Check sheet for the drawn part. Datum: minimum x, y, z corner. Units: mm. A direction names the side the tool comes from. Coordinates: 2 decimals unless noted, no trailing zeros. Order: outer loops, then holes, each group sorted by start corner. A loop starts at its lowest first (then second) coordinate and runs counter-clockwise, first axis right, second up. Notation, with made-up numbers: M 9,22.25 L 44,22.25 A31 cw 44,59.25 Z; hole C 83,78.25 d10. An arc over 180 degrees is marked long. Return JSON: item names as keys, results as strings. Group by question number.
Q1. Section check C-C, the plane x = 30. Enter the section's corners in (y, z), then the cut area to 3 significant figures.
Q2. Access from +Z, -Z, +X, -X, +Y, -Y to the whole of each face (thin tool, end or side, straight path). Record for the marked faces 1 and 2.
Q3. Go/stop test with flat-tipped pins: pin 1 Ø3.5 at (y, z) = (42, 6.5) entering from -X; pin 2 Ø3.5 at (y, z) = (39, 6) entering from +X. Record where each tip stops, or that it passes through.
Q4. Section check D-D, the plane y = 54.5. Enter the section's corners in (x, z), then the cut area to 3 significant figures.
Q5. Thickness scan on probe 1 along X at (y, z) = (22, 1.75); probe 2 along Z at (x, y) = (50, 20); probe 3 along X at (y, z) = (25.5, 8.25). Record the ranges inside material, lowest first.
Q6. Section check B-B, the plane y = 21. Enter the section's corners in (x, z).
Q7. Section check A-A, the plane z = 9. Enter the section's corners in (x, y), then the cut area to 3 significant figures.
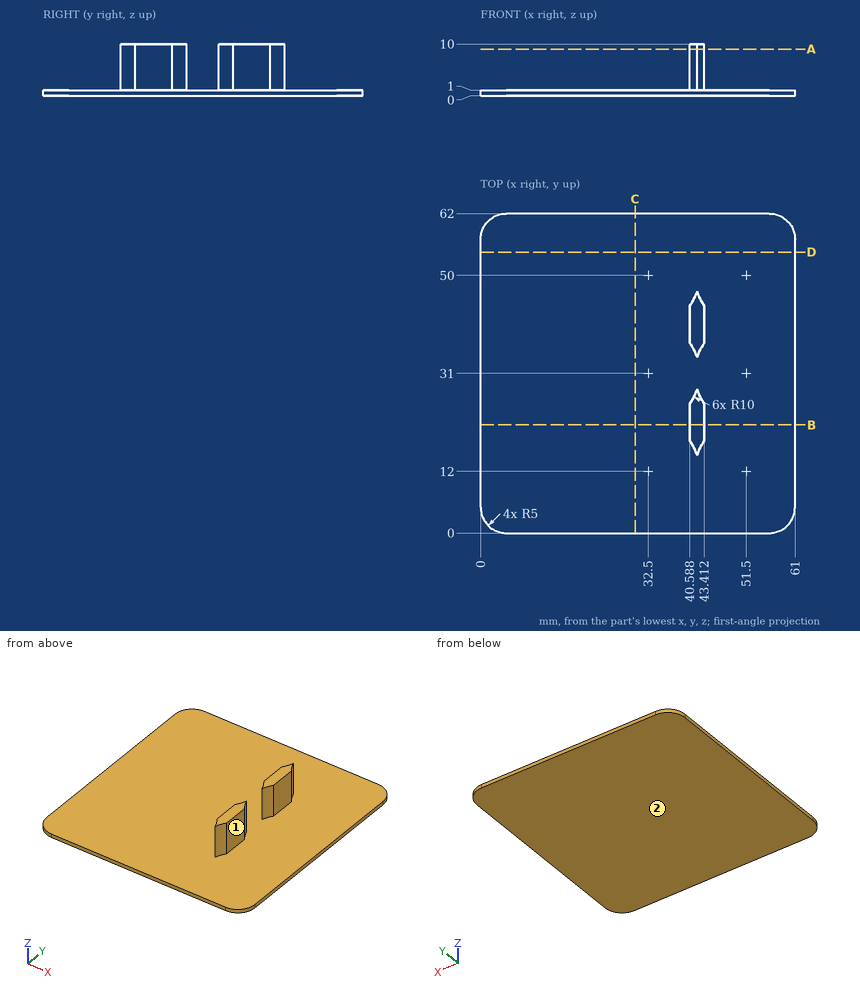
Numbers:
{
 "1": {"outline": "M 0,0 L 62,0 L 62,1 L 0,1 Z", "area": "62.0 mm2"},
 "2": {"face 1": "+Z, +X, +Y, -Y", "face 2": "-Z, +X, -X, +Y, -Y"},
 "3": {"pin 1": "stops at x = 40.59", "pin 2": "stops at x = 43.41"},
 "4": {"outline": "M 0,0 L 61,0 L 61,1 L 0,1 Z", "area": "61.0 mm2"},
 "5": {"probe 1": "x = 40.59 to 43.41", "probe 2": "z = 0 to 1", "probe 3": "x = 40.85 to 43.15"},
 "6": {"outline": "M 0,0 L 61,0 L 61,1 L 43.41,1 L 43.41,10 L 40.59,10 L 40.59,1 L 0,1 Z"},
 "7": {"outline": "M 40.59,17.88 A10 cw 42,15.12 A10 cw 43.41,17.88 L 43.41,25.12 A10 cw 42,27.88 A10 cw 40.59,25.12 Z; M 40.59,36.88 A10 cw 42,34.12 A10 cw 43.41,36.88 L 43.41,44.12 A10 cw 42,46.88 A10 cw 40.59,44.12 Z", "area": "54.5 mm2"}
}
